Source: CAD feature listing. Evaluate the final solid. Frame: model axes, mm. A direction names the side the tool comes from. Give positions to 0.01 mm unless a question says otherwise; leave off trailing zeros. Loops run counter-clockwise (first coordinate to the right, second up) from the corner with the lowest first, then second, coordinate; pieces in that order, holes last. Notation, with made-up numbers: (89.25, 15.5) -> (130.25, 15.5) arc R14 ccw to (130.25, 20.5) -> close; hole circle Ø5 at (72, -8). An arc over 180 degrees is marked (long way). Return JSON: item names as keys, results as strings. Group by question number.
(1) Ray query, line 1 (X direction, y = 3.75, z = -10); line 2 (Z direction, x = 19.5, y = 8.25); line 3 (Z direction, x = 13, y = 4.5). Return the intervals inside material, ascending. Write a range as from..to.
(2) Draft query along Z for faces 1 (the face through (7.19, 5.94, -11.73)), 2 (the face through (37.24, 1.01, -10.99)), 3 (the face through (-6.79, 0.99, -5.07)). Return one class per face: released by +Z, released by -Z, zero draft, split by the parting line, or undercut.
(3) Access query for faces 4 (the face through (15, 0, -10)), 5 (the face through (8, 5, -10)). Directions: +Z, -Z, +X, -X, +Y, -Y. A direction counts if a zero-diameter tool reaches every point of the face in a straight line with its end or side. Return the directions, or none.
(4) Cut plane A-A on y = 1.5. Return loops of the section in (x, z), then the cut area to 3 significant figures.
(5) Cut plane D-D on x = 15. Return loops of the section in (y, z), then the cut area to 3 significant figures.
(6) Cut plane B-B on x = -8. Return loops of the section in (y, z), then the cut area to 3 significant figures.
(7) Cut plane C-C on z = -4. Return loops of the section in (x, y).
(8) Pin query (flat end, axial travel): pin 1 (6 mm diameter, centred on x = 11, z = -10.5, fed in from +Y); pin 2 (11 mm diameter, centred on x = 15, z = -10, fed in from +Y); pin 3 (1.5 mm diameter, centred on x = 20.5, y = 7, fed in from -Z); pin 4 (3 mm diameter, centred on x = 38, z = -10, fed in from +Y). Return the tip coordinate at first contact, or that it passes through.
```python
from build123d import *

# Parameters (mm, degrees)
SKETCH1_W           = 30
SKETCH1_H           = 20
BOSS_EXTRUDE1_DEPTH = 2
SKETCH4_R           = 8
BOSS_EXTRUDE2_DEPTH = 8
SHELL1_START        = 1
SHELL1_OUTLINE_R    = 7
SHELL1_DEPTH        = 9
SKETCH5_R           = 1.25
CUT_EXTRUDE1_DEPTH  = 8
SKETCH6_R           = 1.25
CUT_EXTRUDE2_DEPTH  = 8


# Read off the part's stored shape, not the designer's step: Shell1
with BuildPart() as part:
    # Sketch1 → Boss-Extrude1 (new body)
    with BuildSketch(Plane(origin=(0, 0, 0), x_dir=(1, 0, 0), z_dir=(0, 1, 0))):
        Polygon((30, 0), (43.389820148, 10), (30, 20), align=None)
        Polygon((0, 20), (-13.389820148, 10), (0, 0), align=None)
        with Locations((15, 10)):
            Rectangle(SKETCH1_W, SKETCH1_H)
    extrude(amount=BOSS_EXTRUDE1_DEPTH)

    # Sketch4 → Boss-Extrude2 (add)
    with BuildSketch(Plane(origin=(0, 2, 0), x_dir=(1, 0, 0), z_dir=(0, 1, 0))):
        with Locations(Location((15, 10, 0), (0, 0, 270))):
            Circle(SKETCH4_R)
    extrude(amount=BOSS_EXTRUDE2_DEPTH)

    # Shell1 outline → Shell1 (cut)
    with BuildSketch(Plane(origin=(0, 0, 0), x_dir=(1, 0, 0), z_dir=(0, 1, 0)).offset(SHELL1_START)):
        with Locations((15, 10)):
            Circle(SHELL1_OUTLINE_R)
    extrude(amount=SHELL1_DEPTH, mode=Mode.SUBTRACT)

    # Sketch5 → Cut-Extrude1 (cut)
    with BuildSketch(Plane(origin=(0, 2, 0), x_dir=(1, 0, 0), z_dir=(0, 1, 0))):
        with Locations(Location((-8, 10, 0), (0, 0, 270))):
            Circle(SKETCH5_R)
    extrude(amount=-CUT_EXTRUDE1_DEPTH, mode=Mode.SUBTRACT)

    # Sketch6 → Cut-Extrude2 (cut)
    with BuildSketch(Plane(origin=(0, 2, 0), x_dir=(1, 0, 0), z_dir=(0, 1, 0))):
        with Locations(Location((38, 10, 0), (0, 0, 270))):
            Circle(SKETCH6_R)
    extrude(amount=-CUT_EXTRUDE2_DEPTH, mode=Mode.SUBTRACT)


solid = part.part
```
Answers:
{
 "1": {"line 1": "7..8, 22..23", "line 2": "-16.61..-15.36, -4.64..-3.39", "line 3": "-17.75..-16.71, -3.29..-2.25"},
 "2": {"face 1": "split by the parting line", "face 2": "undercut", "face 3": "released by +Z"},
 "3": {"face 4": "+Z, -Z, +X, -X, -Y", "face 5": "+Y"},
 "4": {"outline": "(-13.39, -10) -> (0, -20) -> (30, -20) -> (43.39, -10) -> (30, 0) -> (0, 0) -> close; hole circle Ø2.5 at (-8, -10); hole circle Ø14 at (15, -10); hole circle Ø2.5 at (38, -10)", "area": "704 mm²"},
 "5": {"outline": "(0, -20) -> (2, -20) -> (2, -18) -> (10, -18) -> (10, -17) -> (1, -17) -> (1, -3) -> (10, -3) -> (10, -2) -> (2, -2) -> (2, 0) -> (0, 0) -> close", "area": "42.0 mm²"},
 "6": {"outline": "(0, -14.03) -> (2, -14.03) -> (2, -11.25) -> (0, -11.25) -> close; (0, -8.75) -> (2, -8.75) -> (2, -5.97) -> (0, -5.97) -> close", "area": "11.1 mm²"},
 "7": {"outline": "(-5.36, 0) -> (35.36, 0) -> (35.36, 2) -> (20.29, 2) -> (20.29, 10) -> (18.61, 10) -> (18.61, 1) -> (11.39, 1) -> (11.39, 10) -> (9.71, 10) -> (9.71, 2) -> (-5.36, 2) -> close"},
 "8": {"pin 1": "y = 10", "pin 2": "y = 1", "pin 3": "z = -16.44", "pin 4": "y = 2"}
}
